Can you work these out from the model? Positions are in its coordinate system, mm. A direction names the side the tool comes from. Round coordinates to 2 decimals unless told otherwise and drop trailing zeros. Write each loop counter-clockwise with the first axis right and the second up, starting at its lowest first coordinate (ties: lowest second). Pieces come first, ordered by that corner, then holes. Notation, with made-up numbers: M 80.25,47.5 L 135.25,47.5 A18 cw 135.25,77.5 Z; hole C 29.5,-31.75 d6. An arc over 180 degrees is marked long. Use one line per item in the form item = value. Start each with the question number.
```python
from build123d import *

# Parameters (mm, degrees)
SKETCH1_W         = 180
SKETCH1_H         = 256
SKETCH1_W_2       = 178
SKETCH1_H_2       = 254
EXTRUSION1_DEPTH  = 101.6
SKETCH2_W         = 180
SKETCH2_H         = 25
SKETCH2_W_2       = 25
SKETCH2_H_2       = 256
EXTRUSION3_DEPTH  = 0.8
EXTRUSION10_REACH = 277.239


with BuildPart() as part:
    # Sketch1 → Extrusion1 (new body)
    with BuildSketch(Plane(origin=(0, 0, 0), x_dir=(-1, 0, 0), z_dir=(0, 1, 0))):
        Rectangle(SKETCH1_W, SKETCH1_H)
        Rectangle(SKETCH1_W_2, SKETCH1_H_2, mode=Mode.SUBTRACT)
    extrude(amount=EXTRUSION1_DEPTH)

    # Sketch2 → Extrusion3 (add)
    with BuildSketch(Plane.XZ):
        with Locations((0, 140.5)):
            Rectangle(SKETCH2_W, SKETCH2_H)
        with Locations((0, -140.5)):
            Rectangle(SKETCH2_W, SKETCH2_H)
        with Locations((102.5, 0)):
            Rectangle(SKETCH2_W_2, SKETCH2_H_2)
        with Locations((-102.5, 0)):
            Rectangle(SKETCH2_W_2, SKETCH2_H_2)
    extrude(amount=-EXTRUSION3_DEPTH)

    # Extrusion10: up to this face of the body (flat: up to its plane)
    extrusion10_end = Plane(part.part.faces().sort_by_distance((-90, 0.4, 140.5))[0])
    # Sketch5 → Extrusion10 (add, up to the picked face)
    with BuildSketch(Plane(origin=(90, 0, 0), x_dir=(0, 0, -1), z_dir=(1, 0, 0)), mode=Mode.PRIVATE) as extrusion10_sk1:
        Polygon((-128, 101.6), (-127.2, 101.6), (-108.627893636, 106.576380902), (-108.681483474, 106.776380902), align=None)
    extrusion10_tool1 = split(extrude(extrusion10_sk1.sketch, amount=-EXTRUSION10_REACH, mode=Mode.PRIVATE), bisect_by=extrusion10_end, keep=Keep.BOTH, mode=Mode.PRIVATE)
    # Sketch5 → Extrusion10 (add, up to the picked face)
    with BuildSketch(Plane(origin=(90, 0, 0), x_dir=(0, 0, -1), z_dir=(1, 0, 0)), mode=Mode.PRIVATE) as extrusion10_sk2:
        Polygon((124.909037356, 101.6), (128, 101.6), (108.681483474, 106.776380902), (108.474428238, 106.003640241), align=None)
    extrusion10_tool2 = split(extrude(extrusion10_sk2.sketch, amount=-EXTRUSION10_REACH, mode=Mode.PRIVATE), bisect_by=extrusion10_end, keep=Keep.BOTH, mode=Mode.PRIVATE)
    add(extrusion10_tool1.solids().sort_by(Axis((90, 104.138519, 118.128746), (-1, 0, 0)))[0])
    add(extrusion10_tool2.solids().sort_by(Axis((90, 104.000199, -117.538406), (-1, 0, 0)))[0])


solid = part.part
```
1. Please list where these lines run through material, in increasing order: line 1 along X through (y, z) = (9.5, -2.5); line 2 along Z through (x, y) = (63, 72); line 3 along Y through (x, z) = (-39, 136).
2. Will these pins go through, and if not, where does the flat tip stop? pin 1 (5 mm diameter, centred on x = 58.5, y = 38, fed in from +Z); pin 2 (6 mm diameter, centred on y = 79, z = -32, fed in from +X); pin 3 (20 mm diameter, centred on x = 10.5, z = -137.5, fed in from +Y).
3. If we section it at C-C (x = 26): List the corners of the cut face in (y, z) for me.
4. Which directions (+Z, -Z, +X, -X, +Y, -Y) give clear straight access to the entire face, cutting with the end or side of a thin tool? Please do faces 4 (the face through (1, 50, -127)), 5 (the face through (90, 43, 2)), 6 (the face through (-1, 0.8, 141)).
5. If we section it at D-D (z = -119): List the corners of the cut face in (x, y) for me.
6. If we section it at A-A (y = 7.5): List the corners of the cut face in (x, z) for me, and give its area (3 significant figures).
7. If we mould it in two halves opening along X, with no side actions, what happens to faces 1 (the face through (-89, 50, -2)), 2 (the face through (-103, 0.8, 2)), 3 (the face through (-90, 55, -2))? For each: pulls with the +X half, pulls with the -X half, needs draft (parallel to the pull), parting line crosses it, or undercut.
8. If we section it at B-B (z = -36): List the corners of the cut face in (x, y) for me, and give its area (3 significant figures).
Model answer:
q1.line_1 = -90 to -89, 89 to 90
q1.line_2 = -128 to -127, 127 to 128
q1.line_3 = 0 to 0.8
q2.pin_1 = 128
q2.pin_2 = 90
q2.pin_3 = 101.73
q3.outline = M 0,-153 L 0.8,-153 L 0.8,-128 L 101.6,-128 L 106.78,-108.68 L 106,-108.47 L 101.6,-124.91 L 101.6,-127 L 0,-127 Z; M 0,127 L 101.6,127 L 101.6,127.2 L 106.58,108.63 L 106.78,108.68 L 101.6,128 L 0.8,128 L 0.8,153 L 0,153 Z
q4.face_4 = -Y
q4.face_5 = +Z, -Z, +X, +Y
q4.face_6 = +Z, +X, -X, +Y
q5.outline = M -115,0 L -89,0 L -89,101.6 L -90,101.6 L -90,0.8 L -115,0.8 Z; M -90,103.18 L 90,103.18 L 90,104.01 L -90,104.01 Z; M 89,0 L 115,0 L 115,0.8 L 90,0.8 L 90,101.6 L 89,101.6 Z
q6.outline = M -90,-128 L 90,-128 L 90,128 L -90,128 Z; hole M -89,-127 L 89,-127 L 89,127 L -89,127 Z
q6.area = 868 mm2
q7.face_1 = undercut
q7.face_2 = needs draft
q7.face_3 = pulls with the -X half
q8.outline = M -115,0 L -89,0 L -89,101.6 L -90,101.6 L -90,0.8 L -115,0.8 Z; M 89,0 L 115,0 L 115,0.8 L 90,0.8 L 90,101.6 L 89,101.6 Z
q8.area = 243 mm2
